Here's how the part is built. I have some questions about the finished solid (model axes, mm). Face numbers are marked on the shaded views. A direction names the side the tool comes from. Round coordinates to 2 decimals unless told otherwise and drop trailing zeros. Loops run counter-clockwise (first coordinate to the right, second up) from the corner with the lowest first, then second, coordinate; pieces in that order, holes last. Notation, with made-up numbers: M -20,13 L 14,13 A15 ccw 14,30 Z; hole C 85,4.5 d4. An arc over 180 degrees is marked long. Use a Markdown table: item, result.
from build123d import *

# Parameters (mm, degrees)
BOSS_EXTRUDE1_DEPTH   = 5.35
FILLET1_R             = 2
FILLET2_R             = 50
FILLET3_R             = 3
CUT_EXTRUDE1_DEPTH    = 120.515289654
CUT_EXTRUDE2_DEPTH    = 8.7
SHELL3_START          = 1
SHELL3_DEPTH          = 4.35
CUT_EXTRUDE3_DEPTH    = 4.35
FILLET6_R             = 1
F_2_CLEARANCE_HOLE1_D = 2.2606


# Read off the part's stored shape, not the designer's step: Shell3
with BuildPart() as part:
    # Sketch1 → Boss-Extrude1 (new, symmetric)
    with BuildSketch(Plane(origin=(0, 0, 0), x_dir=(0, 0, -1), z_dir=(1, 0, 0))):
        with BuildLine():
            Line((0, 0), (8.485281374, -8.485281374))
            Line((8.485281374, -8.485281374), (-12.727922061, -29.69848481))
            Line((-12.727922061, -29.69848481), (-37.462892244, -68.482260413))
            Line((-37.462892244, -68.482260413), (-34.443484132, -83.547139186))
            ThreePointArc((-34.443484132, -83.547139186), (-51.327394218, -100.649341384), (-60.88605591, -78.599767092))
            Line((-60.88605591, -78.599767092), (-29.69848481, -29.69848481))
            Line((-29.69848481, -29.69848481), (0, 0))
        make_face()
        Polygon((-55.587939854, -79.591037977), (-43.982885085, -61.39462065), (-39.741600188, -82.555868301), (-47.296955003, -79.107566033), align=None, mode=Mode.SUBTRACT)
    extrude(amount=BOSS_EXTRUDE1_DEPTH, both=True)

    # Fillet1
    fillet1_edges = [part.edges().sort_by_distance(p)[0] for p in [
        (0, -82.555868301, 39.741600188),
        (0, -61.39462065, 43.982885085),
        (0, -79.591037977, 55.587939854),
    ]]
    fillet(fillet1_edges, radius=FILLET1_R)

    # Fillet2
    fillet2_edges = [part.edges().sort_by_distance(p)[0] for p in [
        (0, -29.69848481, 12.727922061),
        (0, -29.69848481, 29.69848481),
    ]]
    fillet(fillet2_edges, radius=FILLET2_R)

    # Fillet3
    fillet3_edges = [part.edges().sort_by_distance(p)[0] for p in [
        (0, 0, 0),
        (0, -8.485281374, -8.485281374),
    ]]
    fillet(fillet3_edges, radius=FILLET3_R)

    # Sketch2 → Cut-Extrude1 (cut, through all)
    with BuildSketch(Plane(origin=(5.35, 0, 0), x_dir=(0, 0, -1), z_dir=(1, 0, 0))):
        with BuildLine():
            ThreePointArc((3.346446609, -8.838834765), (-0.207139317, -5.141732803), (-4.041965779, -8.546235975))
            ThreePointArc((-4.041965779, -8.546235975), (-2.969848481, -11.455129855), (-0.060954601, -12.527247153))
            ThreePointArc((-0.060954601, -12.527247153), (2.364222862, -11.349550248), (3.346446609, -8.838834765))
        make_face()
    extrude(amount=-CUT_EXTRUDE1_DEPTH, mode=Mode.SUBTRACT)

    # Sketch2<3> → Cut-Extrude2 (cut)
    with BuildSketch(Plane(origin=(5.35, 0, 0), x_dir=(0, 0, -1), z_dir=(1, 0, 0))):
        with BuildLine():
            ThreePointArc((-0.060954601, -12.527247153), (-2.969848481, -11.455129855), (-4.041965779, -8.546235975))
            Line((-4.041965779, -8.546235975), (-11.667353013, -17.673561649))
            ThreePointArc((-11.667353013, -17.673561649), (-11.561195872, -20.046477247), (-9.188280275, -20.152634388))
            Line((-9.188280275, -20.152634388), (-0.060954601, -12.527247153))
        make_face()
    extrude(amount=-CUT_EXTRUDE2_DEPTH, mode=Mode.SUBTRACT)

    # Shell3 outline → Shell3 (cut)
    with BuildSketch(Plane.YZ.offset(SHELL3_START)):
        with BuildLine():
            ThreePointArc((-25.487766305, 11.315546566), (-23.591345049, 15.08737762), (-19.826956258, 16.998529133))
            Line((-19.826956258, 16.998529133), (-27.249508266, 24.421081141))
            ThreePointArc((-27.249508266, 24.421081141), (-31.137049165, 27.906978673), (-35.380230094, 30.949982361))
            Line((-35.380230094, 30.949982361), (-79.675200579, 59.199804797))
            ThreePointArc((-79.675200579, 59.199804797), (-98.683454279, 50.9595792), (-83.940176521, 36.404484299))
            Line((-83.940176521, 36.404484299), (-68.085752059, 39.582138666))
            Line((-68.085752059, 39.582138666), (-33.229363122, 17.351921839))
            ThreePointArc((-33.229363122, 17.351921839), (-29.215798711, 14.516830312), (-25.487766305, 11.315546566))
        make_face()
        with BuildLine():
            ThreePointArc((-78.71831814, 40.510748766), (-80.678728763, 41.229436179), (-80.930811667, 43.302157969))
            Line((-80.930811667, 43.302157969), (-79.107566033, 47.296955003))
            Line((-79.107566033, 47.296955003), (-79.363195628, 51.680706992))
            ThreePointArc((-79.363195628, 51.680706992), (-78.378789867, 53.5220833), (-76.291153896, 53.48338626))
            Line((-76.291153896, 53.48338626), (-65.582774367, 46.653946778))
            ThreePointArc((-65.582774367, 46.653946778), (-64.692320748, 44.599880647), (-66.265170518, 43.006695498))
            Line((-66.265170518, 43.006695498), (-78.71831814, 40.510748766))
        make_face(mode=Mode.SUBTRACT)
    extrude(amount=SHELL3_DEPTH, mode=Mode.SUBTRACT)

    # Sketch3 → Cut-Extrude3 (cut)
    with BuildSketch(Plane.ZY.offset(5.35)):
        with BuildLine():
            Line((16.998529133, -19.826956258), (24.421081141, -27.249508266))
            ThreePointArc((24.421081141, -27.249508266), (27.906978673, -31.137049165), (30.949982361, -35.380230094))
            Line((30.949982361, -35.380230094), (59.199804797, -79.675200579))
            ThreePointArc((59.199804797, -79.675200579), (50.9595792, -98.683454279), (36.404484299, -83.940176521))
            Line((36.404484299, -83.940176521), (39.582138666, -68.085752059))
            Line((39.582138666, -68.085752059), (17.351921839, -33.229363122))
            Line((17.351921839, -33.229363122), (11.315546566, -25.487766305))
            ThreePointArc((11.315546566, -25.487766305), (15.08737762, -23.591345049), (16.998529133, -19.826956258))
        make_face()
    extrude(amount=-CUT_EXTRUDE3_DEPTH, mode=Mode.SUBTRACT)

    # Fillet6
    fillet6_edges = [part.edges().sort_by_distance(p)[0] for p in [
        (5.35, -100.649341384, 51.327394218),
        (5.35, -76.0146998, 35.953188188),
        (5.35, -51.393528511, 26.564281485),
        (-5.35, -18.220948211, 1.250385462),
        (5.35, -18.220948211, 1.250385462),
        (-5.35, -56.45228185, 46.761144692),
        (5.35, -56.45228185, 46.761144692),
        (-5.35, -29.884816473, 29.466437966),
        (5.35, -29.884816473, 29.466437966),
        (-5.35, -29.884816473, 12.495875217),
        (5.35, -29.884816473, 12.495875217),
        (-5.35, -4.242640687, -4.242640687),
        (5.35, -4.242640687, -4.242640687),
        (-5.35, -13.978307524, 13.978307524),
        (-5.35, -1.242640687, 0),
        (-5.35, -8.485281374, -7.242640687),
        (5.35, -13.978307524, 13.978307524),
        (5.35, -1.242640687, 0),
        (5.35, -8.485281374, -7.242640687),
        (-5.35, -51.393528511, 26.564281485),
        (-5.35, -76.0146998, 35.953188188),
        (-5.35, -100.649341384, 51.327394218),
    ]]
    fillet(fillet6_edges, radius=FILLET6_R)

    # #2 Clearance Hole1 (through all)
    with Locations(Plane(origin=(1, -85.089251529, 52.013004842), x_dir=(0, 0, 1), z_dir=(1, 0, 0))):
        with Locations((0, 0), (-6.950460518, 1.300422466), (1.300422466, 6.950460517), (-5.650038052, 8.250882984)):
            Hole(F_2_CLEARANCE_HOLE1_D / 2)


solid = part.part
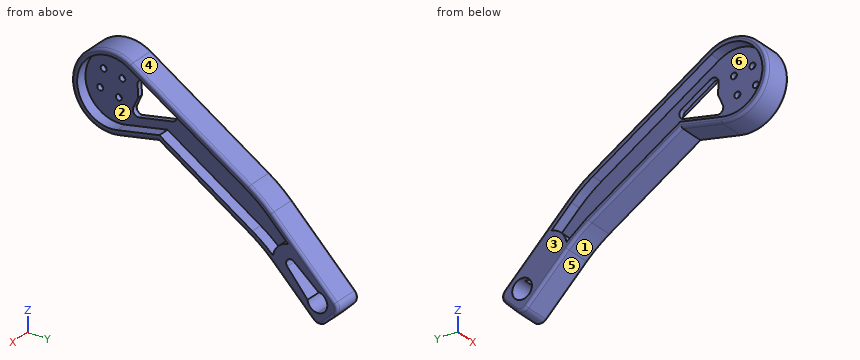
1. Imagine slicing it at A-A, the plane x = -2. Write out the boundary of the cut face in (y, z).
Answer sheet:
| item | result |
|---|---|
| outline | M -83.55,34.44 L -68.48,37.46 L -34.3,15.67 A50 cw -25.84,8.86 L -10.61,-6.36 A3 ccw -6.36,-6.36 L -2.12,-2.12 A3 ccw -2.12,2.12 L -25.84,25.84 A50 ccw -34.3,32.64 L -78.6,60.89 A14.5 ccw long Z; hole M -83.94,36.4 L -68.09,39.58 L -33.23,17.35 L -25.49,11.32 A6.76 cw -19.83,17 L -27.25,24.42 A48 ccw -35.38,30.95 L -79.68,59.2 A12.5 ccw long Z; hole M -20.15,9.19 L -12.53,0.06 A3.7 ccw long -8.55,4.04 L -17.67,11.67 A1.76 ccw Z |
2. Which directions (+Z, -Z, +X, -X, +Y, -Y) give clear straight access to the entire face, cutting with the end or side of a thin tool? Please do the marked faces 1 and 2.
Answer sheet:
| item | result |
|---|---|
| face 1 | -Z, +X, -X, -Y |
| face 2 | +X |
3. I need wall thicknesses on probe 1 along X at (y, z) = (-81, 39); probe 2 along Z at (x, y) = (3.75, -49.5); probe 3 along Y at (x, z) = (-2.25, 30.5). Which ranges of each line are inside material? Lowest first, please. Write a range as from..to.
Answer sheet:
| item | result |
|---|---|
| probe 1 | -1..1 |
| probe 2 | 25.36..27.73, 39.96..42.33 |
| probe 3 | -57.56..-53.85, -34.69..-31.22 |
4. We'd pull the mould along Y, two halves only. Please class the marked faces 3, 4, 5 and 6: +Y half, -Y half, draft (parallel to the pull), parting line (faces both ways), or undercut.
Answer sheet:
| item | result |
|---|---|
| face 3 | draft |
| face 4 | +Y half |
| face 5 | -Y half |
| face 6 | undercut |
5. For pin 1 Ø1.5 at (x, z) = (-2.5, 41.5) entering from -Y; pin 2 Ø1 at (x, z) = (2.5, 30) entering from -Y; pin 3 Ø10 at (y, z) = (-40.5, 15.5) entering from -X; pin 4 Ø1 at (x, z) = (2.5, 9) entering from +Y, each with a flat end and sliding along its axis, tell me the tip position at first contact or that it passes through.
Answer sheet:
| item | result |
|---|---|
| pin 1 | y = -99.4 |
| pin 2 | y = -57.56 |
| pin 3 | x = -5.35 |
| pin 4 | y = -8.5 |
